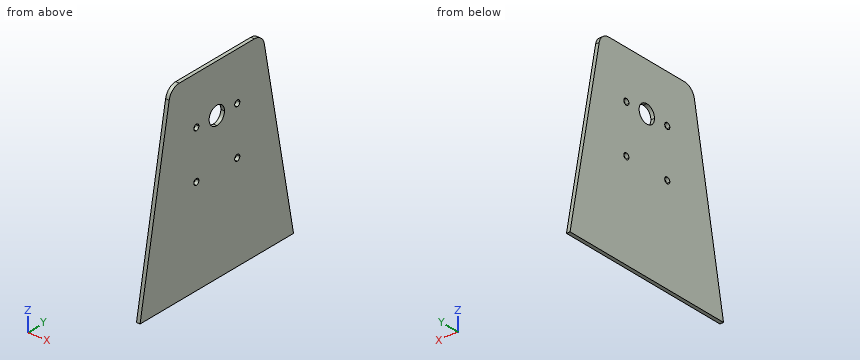
from build123d import *

# Parameters (mm, degrees)
F1_DEPTH = 3
F2_R     = 10


with BuildPart() as f1:
    # F0 (on Right) → F1 (new body)
    with BuildSketch(Plane.YZ):
        Polygon((45, 160), (0, 160), (-45, 160), (-75, 0), (0, 0), (75, 0), align=None)
        with BuildLine():
            ThreePointArc((-20, 82.5), (-18.232233, 81.767767), (-17.5, 80))
            ThreePointArc((-17.5, 80), (-18.232233, 78.232233), (-20, 77.5))
            ThreePointArc((-20, 77.5), (-21.767767, 78.232233), (-22.5, 80))
            ThreePointArc((-22.5, 80), (-21.767767, 81.767767), (-20, 82.5))
        make_face(mode=Mode.SUBTRACT)
        with BuildLine():
            ThreePointArc((-20, 122.5), (-18.232233, 121.767767), (-17.5, 120))
            ThreePointArc((-17.5, 120), (-18.232233, 118.232233), (-20, 117.5))
            ThreePointArc((-20, 117.5), (-21.767767, 118.232233), (-22.5, 120))
            ThreePointArc((-22.5, 120), (-21.767767, 121.767767), (-20, 122.5))
        make_face(mode=Mode.SUBTRACT)
        with BuildLine():
            ThreePointArc((22.5, 80), (21.767767, 78.232233), (20, 77.5))
            ThreePointArc((20, 77.5), (18.232233, 78.232233), (17.5, 80))
            ThreePointArc((17.5, 80), (18.232233, 81.767767), (20, 82.5))
            ThreePointArc((20, 82.5), (21.767767, 81.767767), (22.5, 80))
        make_face(mode=Mode.SUBTRACT)
        with BuildLine():
            ThreePointArc((0, 127.5), (5.303301, 125.303301), (7.5, 120))
            ThreePointArc((7.5, 120), (5.303301, 114.696699), (0, 112.5))
            ThreePointArc((0, 112.5), (-5.303301, 114.696699), (-7.5, 120))
            ThreePointArc((-7.5, 120), (-5.303301, 125.303301), (0, 127.5))
        make_face(mode=Mode.SUBTRACT)
        with BuildLine():
            ThreePointArc((20, 122.5), (21.767767, 121.767767), (22.5, 120))
            ThreePointArc((22.5, 120), (21.767767, 118.232233), (20, 117.5))
            ThreePointArc((20, 117.5), (18.232233, 118.232233), (17.5, 120))
            ThreePointArc((17.5, 120), (18.232233, 121.767767), (20, 122.5))
        make_face(mode=Mode.SUBTRACT)
    extrude(amount=F1_DEPTH)

    # F2
    f2_edges = [f1.edges().sort_by_distance(p)[0] for p in [
        (1.5, -45, 160),
        (1.5, 45, 160),
    ]]
    fillet(f2_edges, radius=F2_R)


solid = f1.part
Model file for the job. Use its own axes, mm. Coordinates: 2 decimals unless noted, no trailing zeros. Write each loop counter-clockwise with the first axis right and the second up, starting at its lowest first coordinate (ties: lowest second). Pieces come first, ordered by that corner, then holes. Notation, with made-up numbers: (42.25, 7.25) -> (71.25, 7.25) arc R26 ccw to (71.25, 25.25) -> close; hole circle Ø3 at (-31, -15). An arc over 180 degrees is marked (long way). One line per item, written item: value. Start each with the question number.
1) Probe probe 1 along Z at (x, y) = (0.35, -18); probe 2 along Z at (x, y) = (2.9, 4.5); probe 3 along Z at (x, y) = (1.9, -6.5). List the from-to ranges inside material, lowest first.
2) Slice it at B-B on y = 53. Write the cut outline in (x, z), then the cut area to 3 significant figures.
3) Slice it at C-C on z = 30.5. Write the cut outline in (x, y).
4) Slice it at A-A on x = 2.5. Write the cut outline in (y, z).
5) Flat gauge pins, fed straight in: pin 1 Ø12 at (y, z) = (-51, 104) entering from -X; pin 2 Ø1 at (x, z) = (1, 63.5) entering from -Y; pin 3 Ø1.5 at (x, z) = (2, 69.5) entering from -Y. Where does each tip first touch, or does it go through?
Answers follow:
1. probe 1: 0 to 78.5, 81.5 to 118.5, 121.5 to 160
1. probe 2: 0 to 114, 126 to 160
1. probe 3: 0 to 116.26, 123.74 to 160
2. outline: (0, 0) -> (3, 0) -> (3, 117.33) -> (0, 117.33) -> close
2. area: 352 mm2
3. outline: (0, -69.28) -> (3, -69.28) -> (3, 69.28) -> (0, 69.28) -> close
4. outline: (-75, 0) -> (75, 0) -> (46.53, 151.84) arc R10 ccw to (36.7, 160) -> (-36.7, 160) arc R10 ccw to (-46.53, 151.84) -> close; hole circle Ø5 at (-20, 80); hole circle Ø5 at (-20, 120); hole circle Ø15 at (0, 120); hole circle Ø5 at (20, 80); hole circle Ø5 at (20, 120)
5. pin 1: x = 0
5. pin 2: y = -63.19
5. pin 3: y = -62.11
